```python
from build123d import *

# Parameters (mm, degrees)
SKETCH_2_R          = 3
CUT_EXTRUDE_1_DEPTH = 15
CUT_EXTRUDE_2_DEPTH = 4


with BuildPart() as part:
    # 草图1 → 旋转1 (revolve)
    with BuildSketch(Plane.XY):
        with BuildLine():
            Line((67.5, 16), (103.5, 16))
            ThreePointArc((103.5, 16), (104.914213562, 16.585786438), (105.5, 18))
            Line((105.5, 18), (105.5, 58))
            Line((105.5, 58), (113.5, 58))
            Line((113.5, 58), (114.5, 50))
            Line((114.5, 50), (142.5, 50))
            Line((142.5, 50), (143.5, 58))
            Line((143.5, 58), (151.5, 58))
            Line((151.5, 58), (151.5, 18))
            ThreePointArc((151.5, 18), (152.085786438, 16.585786438), (153.5, 16))
            Line((153.5, 16), (189.5, 16))
            Line((189.5, 16), (190.5, 15))
            Line((190.5, 15), (190.5, 12.5))
            Line((190.5, 12.5), (285.5, 12.5))
            Line((285.5, 12.5), (286.5, 11.5))
            Line((286.5, 11.5), (286.5, 0))
            Line((286.5, 0), (0, 0))
            Line((0, 0), (0, 11.5))
            Line((0, 11.5), (1, 12.5))
            Line((1, 12.5), (66.5, 12.5))
            Line((66.5, 12.5), (66.5, 15))
            Line((66.5, 15), (67.5, 16))
        make_face()
    revolve(axis=Axis((0, 0, 0), (1, 0, 0)))

    # 草图2 → 切除-拉伸1 (cut, symmetric)
    with BuildSketch(Plane.XY):
        with Locations((256.5, 0)):
            Circle(SKETCH_2_R)
    extrude(amount=CUT_EXTRUDE_1_DEPTH, both=True, mode=Mode.SUBTRACT)

    # 草图3 → 切除-拉伸2 (cut)
    with BuildSketch(Plane.XY.offset(12.5)):
        with BuildLine():
            Line((8, 4), (26, 4))
            ThreePointArc((26, 4), (30, 0), (26, -4))
            Line((26, -4), (8, -4))
            ThreePointArc((8, -4), (4, 0), (8, 4))
        make_face()
    extrude(amount=-CUT_EXTRUDE_2_DEPTH, mode=Mode.SUBTRACT)


solid = part.part
```
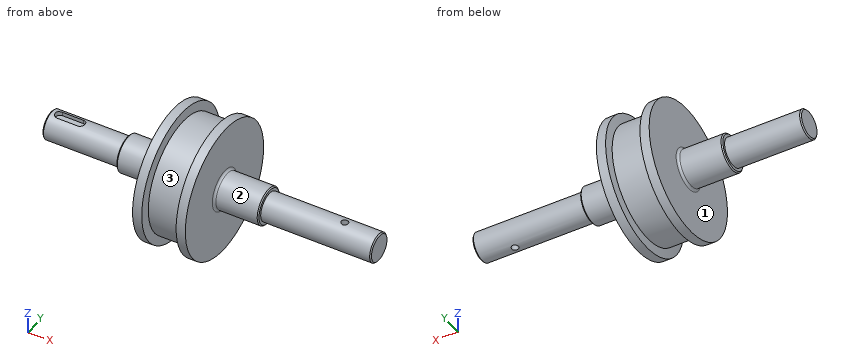
Geometry: final body of the model. Coordinates: model frame, mm. Face numbers are marked on the shaded views. A direction names the side the tool comes from. Coordinates: 2 decimals unless noted, no trailing zeros. Write each loop counter-clockwise with the first axis right and the second up, starting at its lowest first coordinate (ties: lowest second). Pieces come first, ordered by that corner, then holes. Notation, with made-up numbers: M 5.25,76.25 L 42.25,76.25 A11 cw 42.25,88.25 Z; hole C -18,76.25 d6. An arc over 180 degrees is marked long. Answer as CSV lines item,"result". Start each with the question number.
Q1. Cut plane B-B on x = 256.5. Return the cut outline in (y, z).
Q2. Cut plane A-A on x = 100.5. Return the cut outline in (y, z).
Q3. Pin query (flat end, axial travel): P1, Ø1, axis at x = 209.5, y = -7, coming from the -Z side; P2, Ø1, axis at y = -22, z = -24.5, coming from the +X side; P3, Ø2.5, axis at x = 12, y = 1.5, coming from the +Z side; P4, Ø5, axis at x = 256.5, y = 0, coming from the +Z side. Return the tip coordinate at first contact, or that it passes through.
Q4. Line query: line 1 (X direction, y = 0, z = -1); line 2 (X direction, y = 11, z = 36); line 3 (Z direction, x = 162, y = 0). Output: solid intervals per line, ascending. Write a range as from..to.
Q5. Cut plane C-C on x = 43.5. Return the cut outline in (y, z), then the cut area to 3 significant figures.
Q6. Reachability of the marked faces 1, 2 and 3 from +Z, -Z, +X, -X, +Y, -Y: full face, straight path, thin tool, end or side. Return the list, or none.
Findings below:
1,outline,"M -3,-12.13 L -3,12.13 A12.5 ccw Z; M 3,-12.13 A12.5 ccw 3,12.13 Z"
2,outline,"C 0,0 d32"
3,P1,"stops at z = -10.68"
3,P2,"stops at x = 151.5"
3,P3,"stops at z = 8.5"
3,P4,"passes through"
4,line 1,"x = 0..253.5, 259.5..286.5"
4,line 2,"x = 105.5..151.5"
4,line 3,"z = -16..16"
5,outline,"C 0,0 d25"
5,area,"491 mm2"
6,face 1,"-X"
6,face 2,"+X"
6,face 3,"none"
